Here's how the part is built. I have some questions about the finished solid (model axes, mm). A direction names the side the tool comes from. Round coordinates to 2 decimals unless told otherwise and drop trailing zeros. Order: outer loops, then holes, each group sorted by start corner. A loop starts at its lowest first (then second) coordinate and runs counter-clockwise, first axis right, second up. Notation, with made-up numbers: (41.25, 61) -> (71.25, 61) arc R30 cw to (71.25, 88) -> close; hole circle Ø10 at (5, -4). An arc over 180 degrees is marked (long way). Use a Markdown table: item, result. Add a question column.
(1) I want a section at D-D, the plane z = 33. Please give me the cut outline in (x, y), then the cut area to 3 significant figures.
(2) I want a section at A-A, the plane z = -33. Please give me the cut outline in (x, y), then the cut area to 3 significant figures.
(3) If I drill on probe 1 along X at (y, z) = (7.2, -8); probe 2 along Z at (x, y) = (13.5, 5); probe 3 along X at (y, z) = (5.5, -33), over which ranges is the centre line in solid material (lowest first)?
(4) I'm going to push flat-ended pins straight in: P1, Ø1.8, axis at x = -12.5, y = 2.5, coming from the -Z side; P2, Ø2, axis at x = 0, z = -16, coming from the +Y side; P3, Ø3, axis at x = 3.5, z = -15, coming from the -Y side; P4, Ø3, axis at y = 4.5, z = 21, coming from the +X side. Where does each tip first touch, or does it pass through?
(5) I want a section at B-B, the plane x = 8. Please give me the cut outline in (y, z).
(6) On a 3-axis mill with a long thin cutter (end or side, diameter ignored), from which of +Z, -Z, +X, -X, +Y, -Y can I reach the whole of each face in a straight line? I mean faces 1 (the face through (17, 4, 34)), 2 (the face through (17.5, 4, 3)), 3 (the face through (-6, 5.1, 27.2)), 4 (the face through (0, 3, -27)). Say none if no direction works.
(7) Thinking about a two-plate mould opening in Z: for faces 5 (the face through (-0.479, 7.232, -22.845)), 6 (the face through (0, 7, 21)), 7 (the face through (3, 8.5, 0)), which applies, pulls with the +Z half, pulls with the -Z half, needs draft (parallel to the pull), parting line crosses it, or undercut?
(8) I want a section at C-C, the plane y = 4.25. Give the number of separate pieces and of enclosed holes in the cut face, then the cut area to 3 significant figures.
from build123d import *

# Parameters (mm, degrees)
SKETCH1_W                      = 39
SKETCH1_H                      = 62
SKETCH1_W_2                    = 31
SKETCH1_H_2                    = 54
BASE_DEPTH                     = 6
SKETCH2_W                      = 39
SKETCH2_H                      = 62
SKETCH2_R                      = 1.25
TOP_COVER_DEPTH                = 2.5
SKETCH3_R                      = 1.4
MOUNTING_ENDS_DEPTH            = 8.5
BASKET_MOUNTING_EDGE_DEPTH     = 8.5
SKETCH6_R                      = 1.4
BASKET_CLAMP_SCREW_HOLES_DEPTH = 8
SKETCH8_W                      = 12
SKETCH8_H                      = 8.5
USB_OPENING_DEPTH              = 10
F_1MM_EDGE_FILLETS_R           = 1
SKETCH7_W                      = 3
SKETCH7_H                      = 5
ZIP_TIE_HOLE_DEPTH             = 47.954765466


with BuildPart() as part:
    # Sketch1 → Base (new body)
    with BuildSketch(Plane(origin=(0, 0, 0), x_dir=(1, 0, 0), z_dir=(0, 1, 0))):
        Rectangle(SKETCH1_W, SKETCH1_H)
        Rectangle(SKETCH1_W_2, SKETCH1_H_2, mode=Mode.SUBTRACT)
    extrude(amount=BASE_DEPTH)

    # Sketch2 → Top Cover (add)
    with BuildSketch(Plane(origin=(0, 6, 0), x_dir=(1, 0, 0), z_dir=(0, 1, 0))):
        Rectangle(SKETCH2_W, SKETCH2_H)
        with Locations(Location((-12, 24, 0), (0, 0, 270))):
            Circle(SKETCH2_R, mode=Mode.SUBTRACT)
        with Locations(Location((-6, 24, 0), (0, 0, 270))):
            Circle(SKETCH2_R, mode=Mode.SUBTRACT)
        with Locations(Location((0, 24, 0), (0, 0, 270))):
            Circle(SKETCH2_R, mode=Mode.SUBTRACT)
        with Locations(Location((6, 24, 0), (0, 0, 270))):
            Circle(SKETCH2_R, mode=Mode.SUBTRACT)
        with Locations(Location((12, 24, 0), (0, 0, 270))):
            Circle(SKETCH2_R, mode=Mode.SUBTRACT)
        with Locations(Location((-6, 16, 0), (0, 0, 270))):
            Circle(SKETCH2_R, mode=Mode.SUBTRACT)
        with Locations(Location((0, 16, 0), (0, 0, 270))):
            Circle(SKETCH2_R, mode=Mode.SUBTRACT)
        with Locations(Location((6, 16, 0), (0, 0, 270))):
            Circle(SKETCH2_R, mode=Mode.SUBTRACT)
        with Locations(Location((12, 16, 0), (0, 0, 270))):
            Circle(SKETCH2_R, mode=Mode.SUBTRACT)
        with Locations(Location((-6, 8, 0), (0, 0, 270))):
            Circle(SKETCH2_R, mode=Mode.SUBTRACT)
        with Locations(Location((0, 8, 0), (0, 0, 270))):
            Circle(SKETCH2_R, mode=Mode.SUBTRACT)
        with Locations(Location((6, 8, 0), (0, 0, 270))):
            Circle(SKETCH2_R, mode=Mode.SUBTRACT)
        with Locations(Location((12, 8, 0), (0, 0, 270))):
            Circle(SKETCH2_R, mode=Mode.SUBTRACT)
        with Locations(Location((-12, 16, 0), (0, 0, 270))):
            Circle(SKETCH2_R, mode=Mode.SUBTRACT)
        with Locations(Location((-12, 8, 0), (0, 0, 270))):
            Circle(SKETCH2_R, mode=Mode.SUBTRACT)
    extrude(amount=TOP_COVER_DEPTH)

    # Sketch3 → Mounting Ends (add)
    # profile 1 of 2: a face of its own
    with BuildSketch(Plane(origin=(0, 0, 0), x_dir=(1, 0, 0), z_dir=(0, 1, 0))):
        with BuildLine():
            Line((10, 31), (17, 31))
            Line((17, 31), (17, 35))
            ThreePointArc((17, 35), (13.5, 38.5), (10, 35))
            Line((10, 35), (10, 31))
        make_face()
        with Locations(Location((13.5, 33, 0), (0, 0, 90))):
            Circle(SKETCH3_R, mode=Mode.SUBTRACT)
    # profile 2 of 2: a face of its own
    with BuildSketch(Plane(origin=(0, 0, 0), x_dir=(1, 0, 0), z_dir=(0, 1, 0))):
        with BuildLine():
            Line((10, -31), (10, -35))
            ThreePointArc((10, -35), (13.5, -38.5), (17, -35))
            Line((17, -35), (17, -31))
            Line((17, -31), (10, -31))
        make_face()
        with Locations(Location((13.5, -33, 0), (0, 0, 90))):
            Circle(SKETCH3_R, mode=Mode.SUBTRACT)
    extrude(amount=MOUNTING_ENDS_DEPTH)

    # Sketch5 → Basket Mounting Edge (add)
    with BuildSketch(Plane(origin=(0, 0, 0), x_dir=(1, 0, 0), z_dir=(0, 1, 0))):
        with BuildLine():
            Line((19.5, -26), (25.5, -26))
            Line((25.5, -26), (25.5, -24))
            ThreePointArc((25.5, -24), (24.297918472, -23.502081528), (23.8, -22.3))
            Line((23.8, -22.3), (23.8, -19.7))
            ThreePointArc((23.8, -19.7), (24.297918472, -18.497918472), (25.5, -18))
            Line((25.5, -18), (25.5, 1))
            ThreePointArc((25.5, 1), (24.297918472, 1.497918472), (23.8, 2.7))
            Line((23.8, 2.7), (23.8, 5.3))
            ThreePointArc((23.8, 5.3), (24.297918472, 6.502081528), (25.5, 7))
            Line((25.5, 7), (25.5, 9))
            Line((25.5, 9), (19.5, 9))
            Line((19.5, 9), (19.5, -26))
        make_face()
    extrude(amount=BASKET_MOUNTING_EDGE_DEPTH)

    # Sketch6 → Basket Clamp Screw Holes (cut)
    with BuildSketch(Plane(origin=(25.5, 0, 0), x_dir=(0, 0, -1), z_dir=(1, 0, 0))):
        with Locations((-13.5, 4.25)):
            Circle(SKETCH6_R)
        with Locations(Location((-3.5, 4.25, 0), (0, 0, 180))):
            Circle(SKETCH6_R)
    extrude(amount=-BASKET_CLAMP_SCREW_HOLES_DEPTH, mode=Mode.SUBTRACT)

    # Sketch8 → USB Opening (cut)
    with BuildSketch(Plane.XY.offset(31)):
        with Locations((0, 4.25)):
            Rectangle(SKETCH8_W, SKETCH8_H)
    extrude(amount=-USB_OPENING_DEPTH, mode=Mode.SUBTRACT)

    # 1mm Edge Fillets
    f_1mm_edge_fillets_edges = [part.edges().sort_by_distance(p)[0] for p in [
        (19.5, 8.5, -20),
        (19.5, 4.25, -9),
        (19.5, 4.25, 26),
        (22.5, 8.5, -9),
        (22.5, 8.5, 26),
        (-19.5, 8.5, 0),
        (-12.75, 8.5, 31),
        (19.5, 8.5, 28.5),
        (18.25, 8.5, -31),
        (-4.75, 8.5, -31),
        (17, 4.25, -31),
        (10, 4.25, -31),
        (13.5, 8.5, -38.5),
        (10, 8.5, -33),
        (17, 8.5, -33),
        (-19.5, 4.25, -31),
        (19.5, 4.25, -31),
        (19.5, 4.25, 31),
        (-19.5, 4.25, 31),
        (10, 4.25, 31),
        (17, 4.25, 31),
    ]]
    fillet(f_1mm_edge_fillets_edges, radius=F_1MM_EDGE_FILLETS_R)

    # Sketch7 → Zip Tie Hole (cut, through all)
    with BuildSketch(Plane(origin=(0, 8.5, 0), x_dir=(1, 0, 0), z_dir=(0, 1, 0))):
        with Locations((21.5, -8.5)):
            Rectangle(SKETCH7_W, SKETCH7_H)
    extrude(amount=-ZIP_TIE_HOLE_DEPTH, mode=Mode.SUBTRACT)


solid = part.part
Taken from the geometry:
| question | item | result |
|---|---|---|
| 1 | outline | (10, 0) -> (12.1, 0) -> (12.1, 8.5) -> (10, 8.5) -> close; (14.9, 0) -> (17, 0) -> (17, 8.5) -> (14.9, 8.5) -> close |
| 1 | area | 35.7 mm2 |
| 2 | outline | (10, 0) -> (12.1, 0) -> (12.1, 8.5) -> (11, 8.5) arc R1 ccw to (10, 7.5) -> close; (14.9, 0) -> (17, 0) -> (17, 7.5) arc R1 ccw to (16, 8.5) -> (14.9, 8.5) -> close |
| 2 | area | 35.3 mm2 |
| 3 | probe 1 | x = -19.5 to -13.25, -10.75 to -7.25, -4.75 to -1.25, 1.25 to 4.75, 7.25 to 10.75, 13.25 to 25.5 |
| 3 | probe 2 | z = -38.5 to -34.4, -31.6 to -27, 27 to 31.6, 34.4 to 38.5 |
| 3 | probe 3 | x = 10 to 12.1, 14.9 to 17 |
| 4 | P1 | stops at z = -31 |
| 4 | P2 | passes through |
| 4 | P3 | stops at y = 6 |
| 4 | P4 | stops at x = 23.81 |
| 5 | outline | (0, -31) -> (7.5, -31) arc R1 ccw to (8.5, -30) -> (8.5, 31) -> (0, 31) -> (0, 27) -> (6, 27) -> (6, -27) -> (0, -27) -> close |
| 6 | face 1 | +Z, +X, +Y, -Y |
| 6 | face 2 | +X |
| 6 | face 3 | +Z, +Y, -Y |
| 6 | face 4 | -Y |
| 7 | face 5 | undercut |
| 7 | face 6 | pulls with the +Z half |
| 7 | face 7 | needs draft |
| 8 | separate pieces | 1 |
| 8 | enclosed holes | 3 |
| 8 | area | 911 mm2 |
